```python
from build123d import *

# Parameters (mm, degrees)
F0_R     = 1.6
F0_R_2   = 3
F0_R_3   = 2
F1_DEPTH = 2
F2_SIZE  = 1
F3_SIZE  = 1
F4_SIZE  = 1
F5_SIZE  = 1


with BuildPart() as f1:
    # F0 (on Top) → F1 (new body)
    with BuildSketch(Plane.XY):
        with BuildLine():
            ThreePointArc((0, 187.000727), (-7.5, 214.991108), (-15, 187.000727))
            Line((-15, 187.000727), (-15, -186.999273))
            ThreePointArc((-15, -186.999273), (-7.5, -214.989654), (0, -186.999273))
            Line((0, -186.999273), (0, 187.000727))
        make_face()
        with Locations((-14.572135, -207.061108)):
            Circle(F0_R, mode=Mode.SUBTRACT)
        with Locations((-14.57, -192.918972)):
            Circle(F0_R, mode=Mode.SUBTRACT)
        with Locations((-7.5, -199.989654)):
            Circle(F0_R_2, mode=Mode.SUBTRACT)
        with Locations((-0.43, -207.063243)):
            Circle(F0_R, mode=Mode.SUBTRACT)
        with Locations((-0.427865, -192.921108)):
            Circle(F0_R, mode=Mode.SUBTRACT)
        with Locations((-7.5, -150.000727)):
            Circle(F0_R_3, mode=Mode.SUBTRACT)
        with Locations((-7.5, -75.000727)):
            Circle(F0_R_3, mode=Mode.SUBTRACT)
        with Locations((-14.57, 192.918972)):
            Circle(F0_R, mode=Mode.SUBTRACT)
        with Locations((-14.572135, 207.061108)):
            Circle(F0_R, mode=Mode.SUBTRACT)
        with Locations((-7.5, 0.000727)):
            Circle(F0_R_3, mode=Mode.SUBTRACT)
        with Locations((-7.5, 75.000727)):
            Circle(F0_R_3, mode=Mode.SUBTRACT)
        with Locations((-7.5, 150.000727)):
            Circle(F0_R_3, mode=Mode.SUBTRACT)
        with Locations((-7.5, 199.991108)):
            Circle(F0_R_2, mode=Mode.SUBTRACT)
        with Locations((-0.427865, 192.921108)):
            Circle(F0_R, mode=Mode.SUBTRACT)
        with Locations((-0.43, 207.063243)):
            Circle(F0_R, mode=Mode.SUBTRACT)
    extrude(amount=F1_DEPTH)

    # F2
    f2_edges = [f1.edges().sort_by_distance(p)[0] for p in [
        (-16.17, 192.918972, 2),
    ]]
    chamfer(f2_edges, length=F2_SIZE)

    # F3
    f3_edges = [f1.edges().sort_by_distance(p)[0] for p in [
        (-16.172135, 207.061108, 2),
        (-2.03, 207.063243, 2),
        (-2.027865, 192.921108, 2),
    ]]
    chamfer(f3_edges, length=F3_SIZE)

    # F4
    f4_edges = [f1.edges().sort_by_distance(p)[0] for p in [
        (-16.17, -192.918972, 2),
        (-16.172135, -207.061108, 2),
        (-2.03, -207.063243, 2),
        (-2.027865, -192.921108, 2),
    ]]
    chamfer(f4_edges, length=F4_SIZE)

    # F5
    f5_edges = [f1.edges().sort_by_distance(p)[0] for p in [
        (-9.5, 150.000727, 2),
        (-9.5, 75.000727, 2),
        (-9.5, 0.000727, 2),
        (-9.5, -75.000727, 2),
        (-9.5, -150.000727, 2),
    ]]
    chamfer(f5_edges, length=F5_SIZE)


solid = f1.part
```
The listing builds one solid part. Answer for the finished solid, in the listing's coordinates (mm). Give positions to 0.01 mm unless a question says otherwise; leave off trailing zeros. Order: outer loops, then holes, each group sorted by start corner. A loop starts at its lowest first (then second) coordinate and runs counter-clockwise, first axis right, second up. Notation, with made-up numbers: (50, 31.5) -> (60, 31.5) arc R12 cw to (60, 52.5) -> close; hole circle Ø5 at (13, -12.75). An arc over 180 degrees is marked (long way). Answer as CSV lines item,"result". Start each with the question number.
Q1. A cutting plane is placed at A-A (z = 0.4). Count the separate pieces of the cut face and the enclosed holes in it, then the cut area to 3 significant figures.
Q2. Determine the mould class of faces 1 (the cylindrical face through (-6.95, 214.98, 0.99)), 2 (the flat face through (-11, 3, 2)) for opening direction Y: pulls with the +Y half, pulls with the -Y half, needs draft (parallel to the pull), parting line crosses it, or undercut.
Q3. Find the intervals of material crossed by L1, parallel to Y at x = -0.43, z = 0.65; L2, parallel to Y at x = -1.75, z = 1.4; L3, parallel to X at y = 162, z = 0.55, in increasing order.
Q4. A cutting plane is placed at B-B (y = -54.5). Determine the outline of the cut face in (x, z).
Q5. Given pin 1 (5 mm diameter, centred on x = -14.57, y = -192.92, fed in from +Z); pin 2 (1 mm diameter, centred on y = -149, z = 0.5, fed in from -X), each flat-ended and moving along its own axis, determine where each tip first touches the part or whether it passes through.
Results found:
1,separate pieces,"1"
1,enclosed holes,"15"
1,area,"6,800 mm2"
2,face 1,"undercut"
2,face 2,"needs draft"
3,L1,"-213.22 to -208.66, -205.46 to -194.52, -191.32 to 191.32, 194.52 to 205.46, 208.66 to 213.22"
3,L2,"-213.84 to -208.57, -205.56 to -194.42, -191.42 to 191.42, 194.42 to 205.56, 208.57 to 213.85"
3,L3,"-15 to 0"
4,outline,"(-15, 0) -> (0, 0) -> (0, 2) -> (-15, 2) -> close"
5,pin 1,"z = 1.9"
5,pin 2,"x = -15"
